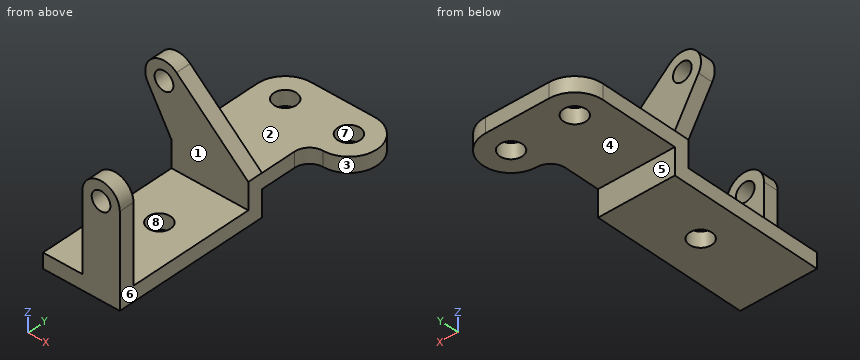
Autodesk Fusion 360 part; units mm, degrees
sketch "Sketch1" plane through (0, 0, 0) normal (0, 0, 1) x (1, 0, 0)
  line L0 (0, 0) -> (82, 0)
  line L1 (82, 0) -> (82, -150)
  line L2 (82, -150) -> (0, -150)
  line L3 (0, -150) -> (0, 0)
  line L4 (0, 0) -> (82, 0)
  line L5 (82, 0) -> (82, 100) construction
  line L6 (82, 100) -> (0, 100) construction
  line L7 (0, 100) -> (0, 0)
  line L8 (0, 16) -> (82, 16)
  line L9 (82, 0) -> (82, 16)
  circle A0 centre (30, 100) radius 12
  circle A1 centre (98, 100) radius 12
  line L10 (30, 130) -> (98, 130)
  line L11 (82, 16) -> (82, 54)
  arc A2 (98, 70) -> (82, 54) centre (98, 54) ccw
  arc A3 (98, 70) -> (98, 130) centre (98, 100) ccw
  arc A4 (30, 130) -> (0, 100) centre (30, 100) ccw
  circle A5 centre (41, -59) radius 12
  dimension "d1" = 150
  dimension "d2" = 82
  dimension "d3" = 82
  dimension "d4" = 100
  dimension "d5" = 16
  dimension "d6" = 24
  dimension "d7" = 24
  dimension "d8" = 30
  dimension "d9" = 98
  dimension "d10" = 60
  dimension "d11" = 60
  dimension "d12" = 32
  dimension "d23" = 24
  dimension "d24" = 41
  dimension "d25" = 59
sketch "Sketch2" plane through (0, 0, 0) normal (0, 1, 0) x (1, 0, 0)
  line L0 (42, -82) -> (82, -82) construction
  line L1 (82, -82) -> (82, 0)
  line L2 (82, 0) -> (42, 0)
  line L3 (42, 0) -> (42, -82)
  circle A0 centre (-8, -82) radius 10
  circle A1 centre (62, -82) radius 10
  line L4 (0, -28) -> (82, -28)
  line L5 (0, -28) -> (-25.3346, -72.0245)
  line L6 (82, -28) -> (5.3693, -96.8748)
  arc A2 (-25.3346, -72.0245) -> (5.3693, -96.8748) centre (-8, -82) ccw
  arc A3 (42, -82) -> (82, -82) centre (62, -82) ccw
  dimension "d26" = 42
  dimension "d27" = 82
  dimension "d28" = 82
  dimension "d29" = 82
  dimension "d30" = 20
  dimension "d31" = 62
  dimension "d32" = 20
  dimension "d33" = 40
  dimension "d34" = 82
  dimension "d35" = 82
  dimension "d36" = 28
  dimension "d38" = 82
  dimension "d39" = 8
extrude "Extrude1" add sketch "Sketch1" against normal blind 16 contours L0 L1 L2 L3 L4
extrude "Extrude2" add sketch "Sketch1" along normal blind 28 and the other way up to surface (16 mm away) contours L0 L4 L7 L8 L9
extrude "Extrude3" add sketch "Sketch1" along normal blind 16 from surface at 12 contours L7 L8 L10 L11 A2 A3 A4
extrude "Extrude5" add sketch "Sketch2" along normal blind 16 from surface at -150 contours L1 L3 L6 A3 | L1 L2 L3 L4 | L3 L4 L6
extrude "Extrude6" add sketch "Sketch2" along normal blind 16 contours L3 L4 L6 | L3 L4 L5 L6 A2
equation "d3 = d2"
equation "d4 = 84 mm + 16 mm"
equation "d9 = d8 + 68 mm"
equation "d25 = 150 mm - 16 mm - 16 mm - 59 mm"
equation "d31 = 42 mm + ( 82 - 42 ) / 2 * 1 mm"
equation "d45 = 28 mm - 16 mm"
Geometry check sheet. Reference: the model listing, model coordinates, mm. Face numbers are marked on the shaded views. A direction names the side the tool comes from. Give positions to 0.01 mm unless a question says otherwise; leave off trailing zeros. Order: outer loops, then holes, each group sorted by start corner. A loop starts at its lowest first (then second) coordinate and runs counter-clockwise, first axis right, second up. Notation, with made-up numbers: (-3, 24.25) - (29, 24.25) arc R27 cw to (29, 60.25) - close; hole circle Ø8 at (18, 28). An arc over 180 degrees is marked (long way). Answer as a JSON object with one key per item and string values.
(1) Cross-section at C-C (x = 106). Record the cut outline in (y, z).
Report:
{"outline": "(71.09, 12) - (91.06, 12) - (91.06, 28) - (71.09, 28) - close; (108.94, 12) - (128.91, 12) - (128.91, 28) - (108.94, 28) - close"}
(2) Cross-section at B-B (y = -59). Record the cut outline in (x, z), then the cut area to 3 significant figures.
Report:
{"outline": "(0, -16) - (29, -16) - (29, 0) - (0, 0) - close; (53, -16) - (82, -16) - (82, 0) - (53, 0) - close", "area": "928 mm^2"}
(3) Material ranges on line 1 (Y direction, x = 44, z = 56.5); line 2 (Y direction, x = 41, z = -6.5); line 3 (Z direction, x = 77.5, y = 76), recorded low to high.
Report:
{"line 1": "-150 to -134, 0 to 16", "line 2": "-150 to -71, -47 to 16", "line 3": "12 to 28"}
(4) Cross-section at A-A (z = 15). Record the cut outline in (x, y).
Report:
{"outline": "(0, 0) - (82, 0) - (82, 54) arc R16 cw to (98, 70) arc R30 ccw to (98, 130) - (30, 130) arc R30 ccw to (0, 100) - close; (42, -150) - (82, -150) - (82, -134) - (42, -134) - close; hole circle Ø24 at (30, 100); hole circle Ø24 at (98, 100)"}
(5) Cross-section at D-D (x = 62). Record the cut outline in (y, z), then the cut area to 3 significant figures.
Report:
{"outline": "(-150, -16) - (16, -16) - (16, 12) - (130, 12) - (130, 28) - (16, 28) - (16, 45.98) - (0, 45.98) - (0, 0) - (-134, 0) - (-134, 72) - (-150, 72) - close; (-150, 92) - (-134, 92) - (-134, 102) - (-150, 102) - close", "area": "6,530 mm^2"}
(6) Tool access check on the marked faces 1, 2, 3 and 4. Record the directions out of +Z, -Z, +X, -X, +Y, -Y that give a thin tool (end or side, any length) a straight path to the whole face; none if there is none.
Report:
{"face 1": "+Z, +X, -X", "face 2": "+Z, +X, -X, +Y", "face 3": "+Z, -Z, +X", "face 4": "-Z, +X, -X, +Y"}
(7) Depth check by flat-ended pin: pin 1 Ø12 at (x, z) = (62, 82) entering from +Y; pin 2 Ø1.5 at (x, z) = (53.5, 69) entering from +Y; pin 3 Ø10 at (x, z) = (7.5, 80) entering from +Y; pin 4 Ø13 at (y, z) = (-139.5, 53.5) entering from -X. Enter the tip coordinate at first touch or a pass-through.
Report:
{"pin 1": "through", "pin 2": "y = -134", "pin 3": "y = 16", "pin 4": "x = 42"}
(8) Draft check along X on the marked faces 5, 6, 7 and 8. Enter one of: released by +X, released by -X, zero draft, split by the parting line, or undercut.
Report:
{"face 5": "zero draft", "face 6": "released by +X", "face 7": "undercut", "face 8": "undercut"}
